Read the model definition and answer for the solid it produces. Units are mm, in the model's axes. Round coordinates to 2 decimals unless told otherwise and drop trailing zeros. Put each result on its own line as item: value.
from build123d import *

# Parameters (mm, degrees)
F0_R      = 2.1
F1_DEPTH  = 20
F1_FACE_R = 2.1
F2_DEPTH  = 204


with BuildPart() as f1:
    # F0 (on Front) → F1 (new body)
    with BuildSketch(Plane.XZ):
        with BuildLine():
            Line((-4.64, 10), (-9, 10))
            ThreePointArc((-9, 10), (-9.707107, 9.707107), (-10, 9))
            Line((-10, 9), (-10, 4.64))
            Line((-10, 4.64), (-8.2, 2.84))
            Line((-8.2, 2.84), (-8.2, 5.49934))
            Line((-8.2, 5.49934), (-6.56, 5.49934))
            Line((-6.56, 5.49934), (-3.90066, 2.84))
            Line((-3.90066, 2.84), (-3.90066, 0.15))
            Line((-3.90066, 0.15), (-3.75066, 0))
            Line((-3.75066, 0), (-3.90066, -0.15))
            Line((-3.90066, -0.15), (-3.90066, -2.84))
            Line((-3.90066, -2.84), (-6.56, -5.49934))
            Line((-6.56, -5.49934), (-8.2, -5.49934))
            Line((-8.2, -5.49934), (-8.2, -2.84))
            Line((-8.2, -2.84), (-10, -4.64))
            Line((-10, -4.64), (-10, -9))
            ThreePointArc((-10, -9), (-9.707107, -9.707107), (-9, -10))
            Line((-9, -10), (-4.64, -10))
            Line((-4.64, -10), (-2.84, -8.2))
            Line((-2.84, -8.2), (-5.49934, -8.2))
            Line((-5.49934, -8.2), (-5.49934, -6.56))
            Line((-5.49934, -6.56), (-2.84, -3.90066))
            Line((-2.84, -3.90066), (-0.15, -3.90066))
            Line((-0.15, -3.90066), (0, -3.75066))
            Line((0, -3.75066), (0.15, -3.90066))
            Line((0.15, -3.90066), (2.84, -3.90066))
            Line((2.84, -3.90066), (5.49934, -6.56))
            Line((5.49934, -6.56), (5.49934, -8.2))
            Line((5.49934, -8.2), (2.84, -8.2))
            Line((2.84, -8.2), (4.64, -10))
            Line((4.64, -10), (9, -10))
            ThreePointArc((9, -10), (9.707107, -9.707107), (10, -9))
            Line((10, -9), (10, -4.64))
            Line((10, -4.64), (8.2, -2.84))
            Line((8.2, -2.84), (8.2, -5.49934))
            Line((8.2, -5.49934), (6.56, -5.49934))
            Line((6.56, -5.49934), (3.90066, -2.84))
            Line((3.90066, -2.84), (3.90066, -0.15))
            Line((3.90066, -0.15), (3.75066, 0))
            Line((3.75066, 0), (3.90066, 0.15))
            Line((3.90066, 0.15), (3.90066, 2.84))
            Line((3.90066, 2.84), (6.56, 5.49934))
            Line((6.56, 5.49934), (8.2, 5.49934))
            Line((8.2, 5.49934), (8.2, 2.84))
            Line((8.2, 2.84), (10, 4.64))
            Line((10, 4.64), (10, 9))
            ThreePointArc((10, 9), (9.707107, 9.707107), (9, 10))
            Line((9, 10), (4.64, 10))
            Line((4.64, 10), (2.84, 8.2))
            Line((2.84, 8.2), (5.49934, 8.2))
            Line((5.49934, 8.2), (5.49934, 6.56))
            Line((5.49934, 6.56), (2.84, 3.90066))
            Line((2.84, 3.90066), (0.15, 3.90066))
            Line((0.15, 3.90066), (0, 3.75066))
            Line((0, 3.75066), (-0.15, 3.90066))
            Line((-0.15, 3.90066), (-2.84, 3.90066))
            Line((-2.84, 3.90066), (-5.49934, 6.56))
            Line((-5.49934, 6.56), (-5.49934, 8.2))
            Line((-5.49934, 8.2), (-2.84, 8.2))
            Line((-2.84, 8.2), (-4.64, 10))
        make_face()
        with BuildLine():
            Line((-8.2, -8.2), (-8.2, -6.71))
            ThreePointArc((-8.2, -6.71), (-8.156066, -6.603934), (-8.05, -6.56))
            Line((-8.05, -6.56), (-7.98749, -6.56))
            Line((-7.98749, -6.56), (-6.603934, -7.943556))
            ThreePointArc((-6.603934, -7.943556), (-6.571418, -7.992219), (-6.56, -8.049622))
            Line((-6.56, -8.049622), (-6.56, -8.05))
            ThreePointArc((-6.56, -8.05), (-6.603934, -8.156066), (-6.71, -8.2))
            Line((-6.71, -8.2), (-8.2, -8.2))
        make_face(mode=Mode.SUBTRACT)
        with BuildLine():
            ThreePointArc((6.71, -8.2), (6.603934, -8.156066), (6.56, -8.05))
            Line((6.56, -8.05), (6.56, -7.98749))
            Line((6.56, -7.98749), (7.943556, -6.603934))
            ThreePointArc((7.943556, -6.603934), (7.992219, -6.571418), (8.049622, -6.56))
            Line((8.049622, -6.56), (8.2, -6.56))
            Line((8.2, -6.56), (8.2, -8.05))
            ThreePointArc((8.2, -8.05), (8.156066, -8.156066), (8.05, -8.2))
            Line((8.05, -8.2), (6.71, -8.2))
        make_face(mode=Mode.SUBTRACT)
        with BuildLine():
            ThreePointArc((-8.2, 8.05), (-8.156066, 8.156066), (-8.05, 8.2))
            Line((-8.05, 8.2), (-6.71, 8.2))
            ThreePointArc((-6.71, 8.2), (-6.603934, 8.156066), (-6.56, 8.05))
            Line((-6.56, 8.05), (-6.56, 8.049622))
            ThreePointArc((-6.56, 8.049622), (-6.571418, 7.992219), (-6.603934, 7.943556))
            Line((-6.603934, 7.943556), (-7.943556, 6.603934))
            ThreePointArc((-7.943556, 6.603934), (-7.992219, 6.571418), (-8.049622, 6.56))
            Line((-8.049622, 6.56), (-8.05, 6.56))
            ThreePointArc((-8.05, 6.56), (-8.156066, 6.603934), (-8.2, 6.71))
            Line((-8.2, 6.71), (-8.2, 8.05))
        make_face(mode=Mode.SUBTRACT)
        Circle(F0_R, mode=Mode.SUBTRACT)
        with BuildLine():
            Line((8.2, 8.05), (8.2, 6.71))
            ThreePointArc((8.2, 6.71), (8.156066, 6.603934), (8.05, 6.56))
            Line((8.05, 6.56), (7.98749, 6.56))
            Line((7.98749, 6.56), (6.56, 7.98749))
            Line((6.56, 7.98749), (6.56, 8.05))
            ThreePointArc((6.56, 8.05), (6.603934, 8.156066), (6.71, 8.2))
            Line((6.71, 8.2), (8.05, 8.2))
            ThreePointArc((8.05, 8.2), (8.156066, 8.156066), (8.2, 8.05))
        make_face(mode=Mode.SUBTRACT)
    extrude(amount=F1_DEPTH)

    # F1_face (on face) → F2 (join)
    with BuildSketch(Plane(origin=(-3.9e-05, -20, 0.000435), x_dir=(1, 0, 0), z_dir=(0, -1, 0))):
        with BuildLine():
            Line((2.840039, 3.900225), (0.150039, 3.900225))
            Line((0.150039, 3.900225), (3.9e-05, 3.750225))
            Line((3.9e-05, 3.750225), (-0.149961, 3.900225))
            Line((-0.149961, 3.900225), (-2.839961, 3.900225))
            Line((-2.839961, 3.900225), (-5.499301, 6.559565))
            Line((-5.499301, 6.559565), (-5.499301, 8.199565))
            Line((-5.499301, 8.199565), (-2.839961, 8.199565))
            Line((-2.839961, 8.199565), (-4.639961, 9.999565))
            Line((-4.639961, 9.999565), (-8.999961, 9.999565))
            ThreePointArc((-8.999961, 9.999565), (-9.707068, 9.706672), (-9.999961, 8.999565))
            Line((-9.999961, 8.999565), (-9.999961, 4.639565))
            Line((-9.999961, 4.639565), (-8.199961, 2.839565))
            Line((-8.199961, 2.839565), (-8.199961, 5.498905))
            Line((-8.199961, 5.498905), (-6.559961, 5.498905))
            Line((-6.559961, 5.498905), (-3.900621, 2.839565))
            Line((-3.900621, 2.839565), (-3.900621, 0.149565))
            Line((-3.900621, 0.149565), (-3.750621, -0.000435))
            Line((-3.750621, -0.000435), (-3.900621, -0.150435))
            Line((-3.900621, -0.150435), (-3.900621, -2.840435))
            Line((-3.900621, -2.840435), (-6.559961, -5.499775))
            Line((-6.559961, -5.499775), (-8.199961, -5.499775))
            Line((-8.199961, -5.499775), (-8.199961, -2.840435))
            Line((-8.199961, -2.840435), (-9.999961, -4.640435))
            Line((-9.999961, -4.640435), (-9.999961, -9.000435))
            ThreePointArc((-9.999961, -9.000435), (-9.707068, -9.707542), (-8.999961, -10.000435))
            Line((-8.999961, -10.000435), (-4.639961, -10.000435))
            Line((-4.639961, -10.000435), (-2.839961, -8.200435))
            Line((-2.839961, -8.200435), (-5.499301, -8.200435))
            Line((-5.499301, -8.200435), (-5.499301, -6.560435))
            Line((-5.499301, -6.560435), (-2.839961, -3.901095))
            Line((-2.839961, -3.901095), (-0.149961, -3.901095))
            Line((-0.149961, -3.901095), (3.9e-05, -3.751095))
            Line((3.9e-05, -3.751095), (0.150039, -3.901095))
            Line((0.150039, -3.901095), (2.840039, -3.901095))
            Line((2.840039, -3.901095), (5.499379, -6.560435))
            Line((5.499379, -6.560435), (5.499379, -8.200435))
            Line((5.499379, -8.200435), (2.840039, -8.200435))
            Line((2.840039, -8.200435), (4.640039, -10.000435))
            Line((4.640039, -10.000435), (9.000039, -10.000435))
            ThreePointArc((9.000039, -10.000435), (9.707146, -9.707542), (10.000039, -9.000435))
            Line((10.000039, -9.000435), (10.000039, -4.640435))
            Line((10.000039, -4.640435), (8.200039, -2.840435))
            Line((8.200039, -2.840435), (8.200039, -5.499775))
            Line((8.200039, -5.499775), (6.560039, -5.499775))
            Line((6.560039, -5.499775), (3.900699, -2.840435))
            Line((3.900699, -2.840435), (3.900699, -0.150435))
            Line((3.900699, -0.150435), (3.750699, -0.000435))
            Line((3.750699, -0.000435), (3.900699, 0.149565))
            Line((3.900699, 0.149565), (3.900699, 2.839565))
            Line((3.900699, 2.839565), (6.560039, 5.498905))
            Line((6.560039, 5.498905), (8.200039, 5.498905))
            Line((8.200039, 5.498905), (8.200039, 2.839565))
            Line((8.200039, 2.839565), (10.000039, 4.639565))
            Line((10.000039, 4.639565), (10.000039, 8.999565))
            ThreePointArc((10.000039, 8.999565), (9.707146, 9.706672), (9.000039, 9.999565))
            Line((9.000039, 9.999565), (4.640039, 9.999565))
            Line((4.640039, 9.999565), (2.840039, 8.199565))
            Line((2.840039, 8.199565), (5.499379, 8.199565))
            Line((5.499379, 8.199565), (5.499379, 6.559565))
            Line((5.499379, 6.559565), (2.840039, 3.900225))
        make_face()
        with BuildLine():
            ThreePointArc((-6.559961, -8.050435), (-6.603895, -8.156501), (-6.709961, -8.200435))
            Line((-6.709961, -8.200435), (-8.199961, -8.200435))
            Line((-8.199961, -8.200435), (-8.199961, -6.710435))
            ThreePointArc((-8.199961, -6.710435), (-8.156027, -6.604369), (-8.049961, -6.560435))
            Line((-8.049961, -6.560435), (-7.987451, -6.560435))
            Line((-7.987451, -6.560435), (-6.603895, -7.943991))
            ThreePointArc((-6.603895, -7.943991), (-6.571379, -7.992654), (-6.559961, -8.050057))
            Line((-6.559961, -8.050057), (-6.559961, -8.050435))
        make_face(mode=Mode.SUBTRACT)
        with BuildLine():
            ThreePointArc((6.710039, -8.200435), (6.603973, -8.156501), (6.560039, -8.050435))
            Line((6.560039, -8.050435), (6.560039, -7.987925))
            Line((6.560039, -7.987925), (7.943595, -6.604369))
            ThreePointArc((7.943595, -6.604369), (7.992258, -6.571853), (8.049661, -6.560435))
            Line((8.049661, -6.560435), (8.200039, -6.560435))
            Line((8.200039, -6.560435), (8.200039, -8.050435))
            ThreePointArc((8.200039, -8.050435), (8.156105, -8.156501), (8.050039, -8.200435))
            Line((8.050039, -8.200435), (6.710039, -8.200435))
        make_face(mode=Mode.SUBTRACT)
        with BuildLine():
            ThreePointArc((-8.049961, 6.559565), (-8.156027, 6.603499), (-8.199961, 6.709565))
            Line((-8.199961, 6.709565), (-8.199961, 8.049565))
            ThreePointArc((-8.199961, 8.049565), (-8.156027, 8.155631), (-8.049961, 8.199565))
            Line((-8.049961, 8.199565), (-6.709961, 8.199565))
            ThreePointArc((-6.709961, 8.199565), (-6.603895, 8.155631), (-6.559961, 8.049565))
            Line((-6.559961, 8.049565), (-6.559961, 8.049187))
            ThreePointArc((-6.559961, 8.049187), (-6.571379, 7.991784), (-6.603895, 7.943121))
            Line((-6.603895, 7.943121), (-7.943517, 6.603499))
            ThreePointArc((-7.943517, 6.603499), (-7.99218, 6.570983), (-8.049583, 6.559565))
            Line((-8.049583, 6.559565), (-8.049961, 6.559565))
        make_face(mode=Mode.SUBTRACT)
        with Locations((3.9e-05, -0.000435)):
            Circle(F1_FACE_R, mode=Mode.SUBTRACT)
        with BuildLine():
            Line((8.200039, 8.049565), (8.200039, 6.709565))
            ThreePointArc((8.200039, 6.709565), (8.156105, 6.603499), (8.050039, 6.559565))
            Line((8.050039, 6.559565), (7.987529, 6.559565))
            Line((7.987529, 6.559565), (6.560039, 7.987055))
            Line((6.560039, 7.987055), (6.560039, 8.049565))
            ThreePointArc((6.560039, 8.049565), (6.603973, 8.155631), (6.710039, 8.199565))
            Line((6.710039, 8.199565), (8.050039, 8.199565))
            ThreePointArc((8.050039, 8.199565), (8.156105, 8.155631), (8.200039, 8.049565))
        make_face(mode=Mode.SUBTRACT)
    extrude(amount=F2_DEPTH)


solid = f1.part
Item 1: Flat-ended cylindrical pins translate along their axes: pin 1 Ø3 at (y, z) = (-143, -1.5) entering from +X; pin 2 Ø2 at (x, y) = (1.5, -65) entering from -Z; pin 3 Ø1 at (x, y) = (1.5, -110.5) entering from +Z. Find the tip coordinate at first contact, or state that the pin passes through.
Derived:
pin 1: stops at x = 8.36
pin 2: stops at z = -3.9
pin 3: stops at z = 3.9
Item 2: The part is cut by section A-A (y = -158.5). State how many separate pieces and enclosed holes the cut face has, then the cut area to 3 significant figures.
Derived:
separate pieces: 1
enclosed holes: 5
area: 164 mm^2
Item 3: Find the intervals of material crossed by line 1 along Z through (x, y) = (0, -178); line 2 along Z through (x, y) = (-7.5, -149); line 3 along Z through (x, y) = (-6.75, -130.5), in increasing order.
Derived:
line 1: z = -3.75 to -2.1, 2.1 to 3.75
line 2: z = -10 to -8.2, -7.05 to -5.5, 5.5 to 7.05, 8.2 to 10
line 3: z = -10 to -8.2, -7.8 to -5.5, 5.5 to 7.8, 8.2 to 10
Item 4: For a pull along Z with two mould halves and no side action, classify faces 1 (the cylindrical face through (2.003, -110.432, 0.631)), 2 (the flat face through (-7, -110, 10)), 3 (the flat face through (-10, -110, -7)) as pulls with the +Z half, pulls with the -Z half, needs draft (parallel to the pull), parting line crosses it, or undercut.
Derived:
face 1: undercut
face 2: pulls with the +Z half
face 3: needs draft
